from build123d import *

# Parameters (mm, degrees)
ESQUISSE1_W             = 34.285714285
ESQUISSE1_H             = 23
ESQUISSE1_W_2           = 25
ESQUISSE1_H_2           = 12
BOSS_EXTRU_1_DEPTH      = 15
ESQUISSE2_W             = 7
ESQUISSE2_H             = 8
ENL_V_MAT_EXTRU_1_DEPTH = 60
ESQUISSE3_R             = 1.1
ENL_V_MAT_EXTRU_2_DEPTH = 10


with BuildPart() as part:
    # Esquisse1 → Boss.-Extru.1 (new body)
    with BuildSketch(Plane(origin=(0, 0, 0), x_dir=(1, 0, 0), z_dir=(0, 1, 0))):
        with Locations((5.428571429, 1.035714286)):
            Rectangle(ESQUISSE1_W, ESQUISSE1_H)
        with Locations((6.142857143, 1.25)):
            Rectangle(ESQUISSE1_W_2, ESQUISSE1_H_2, mode=Mode.SUBTRACT)
    extrude(amount=BOSS_EXTRU_1_DEPTH)

    # Esquisse2 → Enlèv. mat.-Extru.1 (cut)
    with BuildSketch(Plane.ZY.offset(11.714285714)):
        with Locations((-1.035714286, 9)):
            Rectangle(ESQUISSE2_W, ESQUISSE2_H)
    extrude(amount=-ENL_V_MAT_EXTRU_1_DEPTH, mode=Mode.SUBTRACT)

    # Esquisse3 → Enlèv. mat.-Extru.2 (cut)
    with BuildSketch(Plane(origin=(0, 15, 0), x_dir=(1, 0, 0), z_dir=(0, 1, 0))):
        with Locations(Location((-8.857142857, 1.25, 0), (0, 0, 270))):
            Circle(ESQUISSE3_R)
        with Locations(Location((20.071428571, 1.25, 0), (0, 0, 270))):
            Circle(ESQUISSE3_R)
    extrude(amount=-ENL_V_MAT_EXTRU_2_DEPTH, mode=Mode.SUBTRACT)


solid = part.part
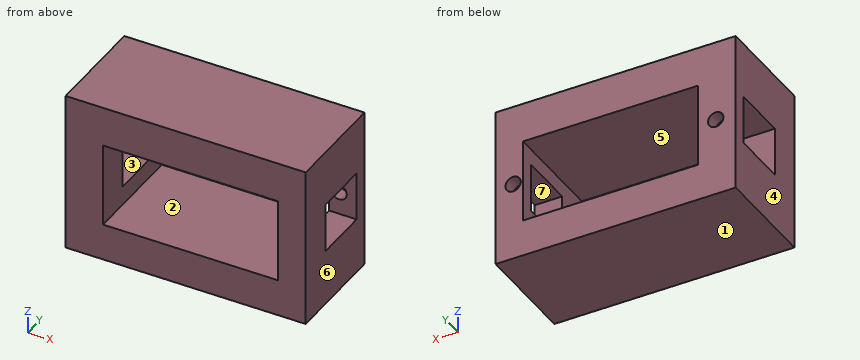
Model file for the job. Use its own axes, mm. Face numbers are marked on the shaded views. A direction names the side the tool comes from. Give positions to 0.01 mm unless a question says otherwise; leave off trailing zeros. Loops run counter-clockwise (first coordinate to the right, second up) from the corner with the lowest first, then second, coordinate; pieces in that order, holes last.
Item 1: Mould opens along X. For the marked faces 4, 5, 6 and 7 say: +X half, -X half, draft (parallel to the pull), parting line (faces both ways), or undercut.
Check values:
face 4: -X half
face 5: undercut
face 6: +X half
face 7: draft
Item 2: Slice it at A-A (y = 10). Write the cut outline in (x, z).
Check values:
outline: (-11.71, -12.54) - (22.57, -12.54) - (22.57, -4.54) - (18.64, -4.54) - (18.64, -7.25) - (-6.36, -7.25) - (-6.36, -4.54) - (-11.71, -4.54) - close; (-11.71, 2.46) - (-6.36, 2.46) - (-6.36, 4.75) - (18.64, 4.75) - (18.64, 2.46) - (22.57, 2.46) - (22.57, 10.46) - (-11.71, 10.46) - close
Item 3: Drill centre lines: line 1 along X through (y, z) = (13.7, -1.25); line 2 along Z through (x, y) = (-0.5, 6); line 3 along X through (y, z) = (1, 2.75). Where is each one in solid material? Low to high.
Check values:
line 1: x = -11.71 to -9.96, -7.76 to -6.36, 18.64 to 18.97, 21.17 to 22.57
line 2: z = -12.54 to -7.25, 4.75 to 10.46
line 3: x = -11.71 to -6.36, 18.64 to 22.57
Item 4: Drop a flat-ended pin along its axis: P1, Ø5, axis at x = 10.5, z = 3, coming from the +Y side. Give the stop position or say it passes through.
Check values:
P1: stops at y = 15
Item 5: Slice it at B-B (z = -1.25). Write the cut outline in (x, y).
Check values:
outline: (-11.71, 0) - (-6.36, 0) - (-6.36, 5) - (-11.71, 5) - close; (-11.71, 13) - (-9.96, 13) - (-9.96, 15) - (-11.71, 15) - close; (-7.76, 13) - (-6.36, 13) - (-6.36, 15) - (-7.76, 15) - close; (18.64, 0) - (22.57, 0) - (22.57, 5) - (18.64, 5) - close; (18.64, 13) - (18.97, 13) - (18.97, 15) - (18.64, 15) - close; (21.17, 13) - (22.57, 13) - (22.57, 15) - (21.17, 15) - close
Item 6: Slice it at C-C (x = 7). Write the cut outline in (y, z), plus the area to 3 significant figures.
Check values:
outline: (0, -12.54) - (15, -12.54) - (15, -7.25) - (0, -7.25) - close; (0, 4.75) - (15, 4.75) - (15, 10.46) - (0, 10.46) - close
area: 165 mm2
Item 7: Which spindle directions (+Z, -Z, +X, -X, +Y, -Y) get a long thin tool onto all of the face, cutting with end or side? Do the marked faces 1, 2 and 3. Say none if no direction does.
Check values:
face 1: -Z, +X, -X, +Y, -Y
face 2: +Y, -Y
face 3: +X, -X
Item 8: Slice it at D-D (z = -4). Write the cut outline in (x, y).
Check values:
outline: (-11.71, 0) - (-6.36, 0) - (-6.36, 5) - (-11.71, 5) - close; (-11.71, 13) - (-6.36, 13) - (-6.36, 15) - (-11.71, 15) - close; (18.64, 0) - (22.57, 0) - (22.57, 5) - (18.64, 5) - close; (18.64, 13) - (22.57, 13) - (22.57, 15) - (18.64, 15) - close
